Input: part model. Units: mm. Frame: model coordinates. A direction names the side the tool comes from. Give positions to 0.01 mm unless a question says otherwise; leave off trailing zeros. Write each loop counter-clockwise with the first axis right and the second up, starting at its lowest first coordinate (ties: lowest second). Pieces come first, ordered by that corner, then holes.
```python
from build123d import *

# Parameters (mm, degrees)
SKETCH1_R             = 6.35
SKETCH1_R_2           = 3.175
BOSS_EXTRUDE1_DEPTH   = 19.05
M4X0_7_TAPPED_HOLE1_D = 3.3
BOSS_EXTRUDE3_DEPTH   = 3.5
FILLET2_R             = 5
SKETCH11_R            = 1.2065
CUT_EXTRUDE1_DEPTH    = 40.736999196
SKETCH12_R            = 3.175
CUT_EXTRUDE2_DEPTH    = 0.635


with BuildPart() as part:
    # Sketch1 → Boss-Extrude1 (new body)
    with BuildSketch(Plane.YZ):
        with Locations(Location((0, 0, 0), (0, 0, 90))):
            Circle(SKETCH1_R)
        with Locations(Location((0, 0, 0), (0, 0, 90))):
            Circle(SKETCH1_R_2, mode=Mode.SUBTRACT)
    extrude(amount=BOSS_EXTRUDE1_DEPTH)

    # M4x0.7 Tapped Hole1 (through all)
    with Locations(Plane(origin=(0, 0, 6.35), x_dir=(0, 1, 0), z_dir=(0, 0, 1))):
        with Locations((0, -15.05)):
            Hole(M4X0_7_TAPPED_HOLE1_D / 2)

    # Sketch10 → Boss-Extrude3 (add)
    with BuildSketch(Plane(origin=(0, 0, 0), x_dir=(0, -1, 0), z_dir=(-1, 0, 0))):
        with BuildLine():
            Line((0, 6.35), (34.29, 6.35))
            Line((34.29, 6.35), (34.29, -6.35))
            Line((34.29, -6.35), (0, -6.35))
            ThreePointArc((0, -6.35), (6.35, 0), (0, 6.35))
        make_face()
    extrude(amount=-BOSS_EXTRUDE3_DEPTH)

    # Fillet2
    fillet2_edges = [part.edges().sort_by_distance(p)[0] for p in [
        (1.75, -34.29, -6.35),
        (1.75, -34.29, 6.35),
    ]]
    fillet(fillet2_edges, radius=FILLET2_R)

    # Sketch11 → Cut-Extrude1 (cut, through all)
    with BuildSketch(Plane(origin=(0, 0, 0), x_dir=(0, -1, 0), z_dir=(-1, 0, 0))):
        with Locations(Location((30.099, 0, 0), (0, 0, 90))):
            Circle(SKETCH11_R)
        with Locations(Location((20.193, 0, 0), (0, 0, 90))):
            Circle(SKETCH11_R)
    extrude(amount=-CUT_EXTRUDE1_DEPTH, mode=Mode.SUBTRACT)

    # Sketch12 → Cut-Extrude2 (cut)
    with BuildSketch(Plane.YZ.offset(3.5)):
        with Locations(Location((-20.193, 0, 0), (0, 0, 270))):
            Circle(SKETCH12_R)
        with Locations(Location((-30.099, 0, 0), (0, 0, 270))):
            Circle(SKETCH12_R)
    extrude(amount=-CUT_EXTRUDE2_DEPTH, mode=Mode.SUBTRACT)


solid = part.part
```
Q1. Section D-D, the plane z = 5.5. Return the cut outline in (x, y).
Q2. Pin query (flat end, axial travel): pin 1 (7 mm diameter, centred on y = -19, z = 1, fed in from +X); pin 2 (3 mm diameter, centred on y = -30, z = 0.5, fed in from +X) (3 decimals); pin 3 (1 mm diameter, centred on x = 6.5, z = -3.5, fed in from -Y). Return the tip coordinate at first contact, or that it passes through.
Q3. Material intervals for line 1 along Y through (x, z) = (3.3, 0) (3 decimals); line 2 along Y through (x, z) = (1.75, 1); line 3 along X through (y, z) = (-24, 2.75), sorted ascending.
Q4. Section C-C, the plane z = 2.25. Return the cut outline in (x, y) (3 decimals).
Q5. Section A-A, the plane z = 0. Give the number of separate pieces and of enclosed holes in the cut face, then the cut area to 3 significant figures.
Q6. Section B-B, the plane x = 15.05. Return the cut outline in (y, z) (3 decimals).
Q7. Access query for faces 4 (the flat face through (2, -34.29, 0)), 5 (the flat face through (2.865, -30.1, -1.4)). Directions: +Z, -Z, +X, -X, +Y, -Y. A direction counts if a zero-diameter tool reaches every point of the face in a straight line with its end or side. Return the directions, or none.
Q8. Mould query, pull axis Z, two halves, no side actions, for faces 1 (the flat face through (3.5, -17, 2)), 2 (the cylindrical face through (1.77, -32.79, 4.92)), 3 (the cylindrical face through (3.19, -33.2, 0.69)). Classes: +Z half, -Z half, draft (parallel to the pull), parting line (faces both ways), or undercut.
Solutions:
1. outline: (0, -32.08) - (3.5, -32.08) - (3.5, -3.17) - (19.05, -3.17) - (19.05, 3.17) - (0, 3.17) - close; hole circle Ø3.3 at (15.05, 0)
2. pin 1: stops at x = 3.5
2. pin 2: stops at x = 2.865
2. pin 3: stops at y = -5.6
3. line 1: y = -34.29 to -33.274, -26.924 to -23.368, -17.018 to -3.175, 3.175 to 6.35
3. line 2: y = -34.29 to -30.77, -29.42 to -20.87, -19.52 to -3.01, 3.01 to 6.27
3. line 3: x = 0 to 3.5
4. outline: (0, -34.208) - (3.5, -34.208) - (3.5, -32.339) - (2.865, -32.339) - (2.865, -27.859) - (3.5, -27.859) - (3.5, -22.433) - (2.865, -22.433) - (2.865, -17.953) - (3.5, -17.953) - (3.5, -5.938) - (19.05, -5.938) - (19.05, -2.24) - (0, -2.24) - close; (0, 2.24) - (19.05, 2.24) - (19.05, 5.938) - (0, 5.938) - close
5. separate pieces: 4
5. enclosed holes: 0
5. area: 197 mm2
6. outline: (-1.65, -6.132) - (-1.65, -2.713) arc R3.175 cw to (-1.65, 2.713) - (-1.65, 6.132) arc R6.35 ccw to start; (1.65, -6.132) arc R6.35 ccw to (1.65, 6.132) - (1.65, 2.713) arc R3.175 cw to (1.65, -2.713) - close
7. face 4: +Z, -Z, +X, -X, -Y
7. face 5: +X
8. face 1: draft
8. face 2: +Z half
8. face 3: undercut
